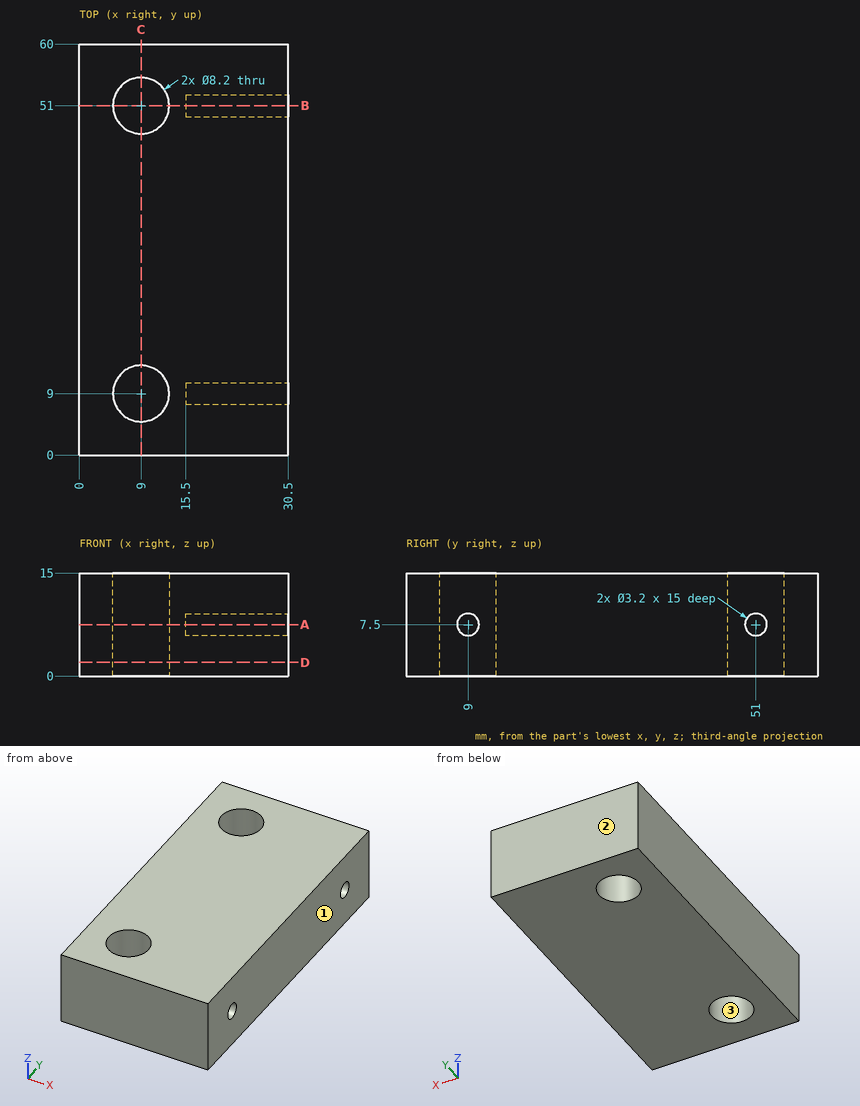
Geometry check sheet. Reference: drawing and pictorial views, mm from the part's lowest x, y, z. Coordinates: 2 decimals unless noted, no trailing zeros. Order: outer loops, then holes, each group sorted by start corner. A loop starts at its lowest first (then second) coordinate and runs counter-clockwise, first axis right, second up. Notation, with made-up numbers: M -33.5,85 L -23.5,85 A17 ccw -23.5,92 Z; hole C 87,50 d3. An arc over 180 degrees is marked long. Return JSON: item names as keys, results as strings.
1) Cross-section at D-D, the plane z = 2. Record the boundary of the cut face in (x, y).
Answer list:
{"outline": "M 0,0 L 30.5,0 L 30.5,60 L 0,60 Z; hole C 9,9 d8.2; hole C 9,51 d8.2"}
2) Release check for a two-part mould opening along X. For the marked faces 1, 2 and 3 record: +X half, -X half, draft (parallel to the pull), parting line (faces both ways), or undercut.
Answer list:
{"face 1": "+X half", "face 2": "draft", "face 3": "undercut"}
3) Thickness scan on L1, parallel to Y at x = 9, z = 5.25; L2, parallel to Y at x = 6, z = 2.5; L3, parallel to X at y = 6, z = 7. Record the ranges inside material, lowest first. Write a range as [from, to].
Answer list:
{"L1": "[0, 4.9], [13.1, 46.9], [55.1, 60]", "L2": "[0, 6.21], [11.79, 48.21], [53.79, 60]", "L3": "[0, 6.21], [11.79, 30.5]"}
4) Cross-section at B-B, the plane y = 51. Record the boundary of the cut face in (x, z), and give its area (4 significant figures).
Answer list:
{"outline": "M 0,0 L 4.9,0 L 4.9,15 L 0,15 Z; M 13.1,0 L 30.5,0 L 30.5,5.9 L 15.5,5.9 L 15.5,9.1 L 30.5,9.1 L 30.5,15 L 13.1,15 Z", "area": "286.5 mm2"}
5) Cross-section at C-C, the plane x = 9. Record the boundary of the cut face in (y, z), and give its area (3 significant figures).
Answer list:
{"outline": "M 0,0 L 4.9,0 L 4.9,15 L 0,15 Z; M 13.1,0 L 46.9,0 L 46.9,15 L 13.1,15 Z; M 55.1,0 L 60,0 L 60,15 L 55.1,15 Z", "area": "654 mm2"}
6) Gauge pin test, flat ends, axial feed: pin 1 (1.9 mm diameter, centred on y = 51, z = 7.5, fed in from +X); pin 2 (6.5 mm diameter, centred on x = 9, y = 9, fed in from +Z). Record the tip position at first contact, or that the pin passes through.
Answer list:
{"pin 1": "x = 15.5", "pin 2": "through"}
7) Cross-section at A-A, the plane z = 7.5. Record the boundary of the cut face in (x, y), and give its area (3 significant figures).
Answer list:
{"outline": "M 0,0 L 30.5,0 L 30.5,7.4 L 15.5,7.4 L 15.5,10.6 L 30.5,10.6 L 30.5,49.4 L 15.5,49.4 L 15.5,52.6 L 30.5,52.6 L 30.5,60 L 0,60 Z; hole C 9,9 d8.2; hole C 9,51 d8.2", "area": "1,630 mm2"}
